Source: CAD feature listing. Evaluate the final solid. Frame: model axes, mm. Face numbers are marked on the shaded views. Give positions to 0.01 mm unless a question says otherwise; leave off trailing zeros. Order: outer loops, then holes, each group sorted by start corner. A loop starts at its lowest first (then second) coordinate and runs counter-clockwise, first axis right, second up.
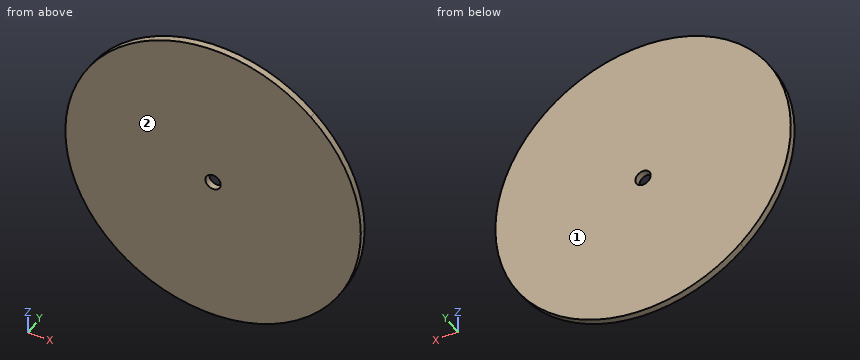
```python
from build123d import *

# Parameters (mm, degrees)
F1_DEPTH = 3.556
F2_D     = 7.9248


with BuildPart() as f1:
    # F0 (on Front) → F1 (new body)
    with BuildSketch(Plane.XZ):
        with BuildLine():
            ThreePointArc((49.052849, -58.590001), (69.236021, -32.331775), (76.413155, 0))
            ThreePointArc((76.413155, 0), (69.662719, 31.401845), (50.604095, 57.255531))
            Line((50.604095, 57.255531), (0.166721, -0.151271))
            Line((0.166721, -0.151271), (49.052849, -58.590001))
        make_face()
        with BuildLine():
            Line((0.166721, -0.151271), (50.604095, 57.255531))
            ThreePointArc((50.604095, 57.255531), (1.053942, 76.405886), (-49.005576, 58.629547))
            Line((-49.005576, 58.629547), (0.166721, -0.151271))
        make_face()
        with BuildLine():
            ThreePointArc((-50.265902, -57.552666), (-0.798054, -76.408988), (49.052849, -58.590001))
            Line((49.052849, -58.590001), (0.166721, -0.151271))
            Line((0.166721, -0.151271), (-50.265902, -57.552666))
        make_face()
        with BuildLine():
            Line((0.166721, -0.151271), (-49.005576, 58.629547))
            ThreePointArc((-49.005576, 58.629547), (-76.40866, 0.828868), (-50.265902, -57.552666))
            Line((-50.265902, -57.552666), (0.166721, -0.151271))
        make_face()
    extrude(amount=F1_DEPTH)

    # F2 (through all)
    with Locations(Plane(origin=(0, 0, 0), x_dir=(1, 0, 0), z_dir=(0, 1, 0))):
        with Locations((0, 0)):
            Hole(F2_D / 2)


solid = f1.part
```
1) Draft query along Y for the marked faces 1 and 2. Return one class per face: +Y half, -Y half, draft (parallel to the pull), parting line (faces both ways), or undercut.
Report:
face 1: +Y half
face 2: -Y half
2) Section query A-A, the plane x = 0. Return the cut outline in (y, z), and give its area (3 significant figures).
Report:
outline: (-3.56, -76.41) - (0, -76.41) - (0, -3.96) - (-3.56, -3.96) - close; (-3.56, 3.96) - (0, 3.96) - (0, 76.41) - (-3.56, 76.41) - close
area: 515 mm2
3) Section query D-D, the plane x = 66. Return the cut outline in (y, z), and give its area (3 significant figures).
Report:
outline: (-3.56, -38.51) - (0, -38.51) - (0, 38.51) - (-3.56, 38.51) - close
area: 274 mm2
4) Material intervals for L1, parallel to Z at x = 0, y = -0.75; L2, parallel to X at y = -1.85, z = 13.5; L3, parallel to X at y = -3, z = 5, sorted ascending.
Report:
L1: z = -76.41 to -3.96, 3.96 to 76.41
L2: x = -75.21 to 75.21
L3: x = -76.25 to 76.25
5) Section query C-C, the plane z = 25. Return the cut outline in (x, y).
Report:
outline: (-72.21, -3.56) - (72.21, -3.56) - (72.21, 0) - (-72.21, 0) - close
6) Section query B-B, the plane y = -2.1. Return the cut outline in (x, z).
Report:
outline: (-50.27, -57.55) arc R76.41 ccw to (49.05, -58.59) arc R76.41 ccw to (76.41, 0) arc R76.41 ccw to (50.6, 57.26) arc R76.41 ccw to (-49.01, 58.63) arc R76.41 ccw to start; hole circle Ø7.92 at (0, 0)
7) Pin query (flat end, axial travel): pin 1 (7 mm diameter, centred on x = 0, z = 0, fed in from -Y); pin 2 (5 mm diameter, centred on x = 37.5, z = 10.5, fed in from +Y). Return the tip coordinate at first contact, or that it passes through.
Report:
pin 1: passes through
pin 2: stops at y = 0
